Part print with two shaded views. Sizes in mm from the minimum x, y, z corner. A direction names the side the tool comes from. Coordinates: 2 decimals unless noted, no trailing zeros. Write each loop counter-clockwise with the first axis right and the second up, starting at its lowest first coordinate (ties: lowest second). Pieces come first, ordered by that corner, then holes.
Q1. Drill centre lines: probe 1 along X at (y, z) = (5.5, 3.5); probe 2 along Y at (x, z) = (5, 3.95); probe 3 along Y at (x, z) = (14.5, 2.8). Where is each one in solid material? Low to high.
Q2. Band-saw the part on D-D, the plane x = 14.5. Write the cut outline in (y, z).
Q3. Band-saw the part on B-B, the plane z = 4.35. Write the cut outline in (x, y), plus the area to 3 significant figures.
Q4. Pin check, flat tips, straight feed: P1, Ø1.5, axis at x = 20, z = 1.5, coming from the +Y side; P2, Ø2, axis at x = 36.5, y = 3, coming from the -Z side; P3, Ø1, axis at y = 7, z = 5, coming from the +X side. Stop position of each tip, or through.
Q5. Band-saw the part on C-C, the plane y = 6. State how many separate pieces and enclosed holes the cut face has, plus the area to 3 significant figures.
Q6. Which spindle directions (+Z, -Z, +X, -X, +Y, -Y) get a long thin tool onto all of the face, cutting with end or side? Do the marked faces 1 and 2. Say none if no direction does.
Q7. Pull direction Y, two halves, no side cores. Call the marked faces 3, 4 and 5: released by +Y, released by -Y, zero draft, split by the parting line, or undercut.
Q8. Band-saw the part on A-A, the plane x = 37. Write the cut outline in (y, z).
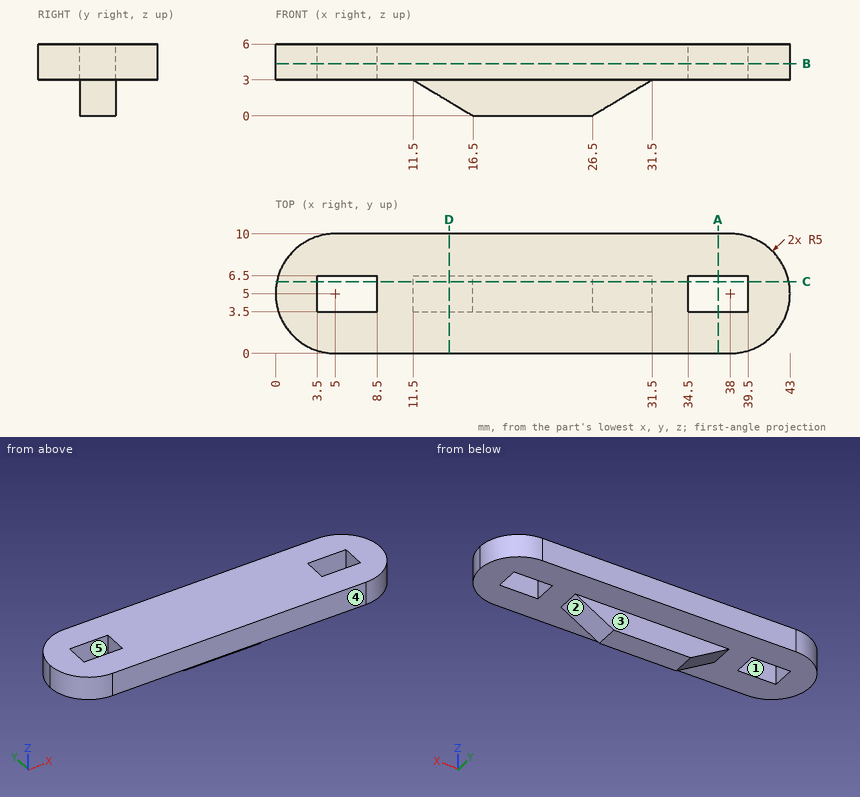
Answer sheet:
1. probe 1: x = 0.03 to 3.5, 8.5 to 34.5, 39.5 to 42.97
1. probe 2: y = 0 to 3.5, 6.5 to 10
1. probe 3: y = 3.5 to 6.5
2. outline: (0, 3) - (3.5, 3) - (3.5, 1.2) - (6.5, 1.2) - (6.5, 3) - (10, 3) - (10, 6) - (0, 6) - close
3. outline: (5, 0) - (38, 0) arc R5 ccw to (38, 10) - (5, 10) arc R5 ccw to start; hole (3.5, 3.5) - (8.5, 3.5) - (8.5, 6.5) - (3.5, 6.5) - close; hole (34.5, 3.5) - (39.5, 3.5) - (39.5, 6.5) - (34.5, 6.5) - close
3. area: 379 mm2
4. P1: stops at y = 6.5
4. P2: stops at z = 3
4. P3: stops at x = 42.77
5. separate pieces: 3
5. enclosed holes: 0
5. area: 143 mm2
6. face 1: +Z, -Z
6. face 2: -Z, +X, +Y, -Y
7. face 3: released by +Y
7. face 4: released by -Y
7. face 5: undercut
8. outline: (0, 3) - (3.5, 3) - (3.5, 6) - (0, 6) - close; (6.5, 3) - (10, 3) - (10, 6) - (6.5, 6) - close
